Part model, mm, in its own coordinate system. Face numbers are marked on the shaded views. A direction names the side the tool comes from. Coordinates: 2 decimals unless noted, no trailing zeros. Write each loop counter-clockwise with the first axis right and the second up, starting at its lowest first coordinate (ties: lowest second). Pieces come first, ordered by that corner, then holes. Notation, with made-up numbers: M -6.5,33.25 L 6.5,33.25 A7 cw 6.5,45.25 Z; hole C 49,78.25 d3. An arc over 180 degrees is marked long. Use a Markdown table: item, result. Add a question column.
Q1. Slice it at B-B on y = 5. Write the cut outline in (x, z).
Q2. Slice it at D-D on x = 1.5. Write the cut outline in (y, z), then the cut area to 3 significant figures.
Q3. Tool access for the marked faces 1, 2 and 3: list every direction of +Z, -Z, +X, -X, +Y, -Y with a clear straight run to the whole face (end or side of a thin tool).
Q4. Pin check, flat tips, straight feed: pin 1 Ø2 at (x, y) = (16, 5) entering from +Z; pin 2 Ø11 at (x, y) = (14.5, 6) entering from -Z; pin 3 Ø2 at (x, z) = (8.5, 9.5) entering from +Y; pin 4 Ø5 at (y, z) = (6, 14) entering from +X. Stop position of each tip, or through.
Q5. Slice it at C-C on z = 7.25. Write the cut outline in (x, y).
Q6. Wall check: L1, parallel to Y at x = 24.5, z = 23.45; L2, parallel to Y at x = 21, z = 19.75; L3, parallel to X at y = 9, z = 18.5. Give the ranges that are in metal, low to high. Write a range as from..to.
Q7. Slice it at A-A on x = 16. Write the cut outline in (y, z).
from build123d import *

# Parameters (mm, degrees)
SKETCH1_W           = 12.5
SKETCH1_H           = 10
BOSS_EXTRUDE1_DEPTH = 10
SKETCH2_W           = 10
SKETCH2_H           = 10
BOSS_EXTRUDE2_DEPTH = 5
SKETCH3_R           = 3.75
BOSS_EXTRUDE3_DEPTH = 17
SKETCH4_W           = 4
SKETCH4_H           = 10
CUT_EXTRUDE1_DEPTH  = 11
SKETCH5_W           = 9.5
SKETCH5_H           = 10
BOSS_EXTRUDE4_DEPTH = 12.5
SKETCH6_W           = 5
SKETCH6_H           = 10
BOSS_EXTRUDE5_DEPTH = 30
SKETCH7_R           = 1.75
CUT_EXTRUDE2_DEPTH  = 23.5
SKETCH8_W           = 30
SKETCH8_H           = 5
CUT_EXTRUDE4_DEPTH  = 10
SKETCH10_W          = 9.5
SKETCH10_H          = 10
CUT_EXTRUDE6_DEPTH  = 3.49
SKETCH11_W          = 9.5
SKETCH11_H          = 10
BOSS_EXTRUDE6_DEPTH = 3.9
SKETCH12_W          = 4
SKETCH12_H          = 10
BOSS_EXTRUDE7_DEPTH = 20
SKETCH13_W          = 20
SKETCH13_H          = 0.09
CUT_EXTRUDE7_DEPTH  = 28
SKETCH14_R          = 1.75
CUT_EXTRUDE8_DEPTH  = 23.91
SKETCH15_W          = 29.5
SKETCH15_H          = 10
SKETCH15_R          = 1.75
BOSS_EXTRUDE8_DEPTH = 1
FILLET1_R           = 2


with BuildPart() as part:
    # Sketch1 → Boss-Extrude1 (new body)
    with BuildSketch(Plane.XY):
        with Locations((6.25, 5)):
            Rectangle(SKETCH1_W, SKETCH1_H)
    extrude(amount=BOSS_EXTRUDE1_DEPTH)

    # Sketch2 → Boss-Extrude2 (add)
    with BuildSketch(Plane.ZY):
        with Locations((5, 5)):
            Rectangle(SKETCH2_W, SKETCH2_H)
    extrude(amount=BOSS_EXTRUDE2_DEPTH)

    # Sketch3 → Boss-Extrude3 (add)
    with BuildSketch(Plane(origin=(0, 10, 0), x_dir=(1, 0, 0), z_dir=(0, 1, 0))):
        with Locations((3.75, -5)):
            Circle(SKETCH3_R)
    extrude(amount=BOSS_EXTRUDE3_DEPTH)

    # Sketch4 → Cut-Extrude1 (cut, through all)
    with BuildSketch(Plane(origin=(0, 10, 0), x_dir=(1, 0, 0), z_dir=(0, 1, 0))):
        with Locations((10.5, -5)):
            Rectangle(SKETCH4_W, SKETCH4_H)
        with Locations((-3, -5)):
            Rectangle(SKETCH4_W, SKETCH4_H)
    extrude(amount=-CUT_EXTRUDE1_DEPTH, mode=Mode.SUBTRACT)

    # Sketch5 → Boss-Extrude4 (add)
    with BuildSketch(Plane.XY.offset(10)):
        with Locations((3.75, 5)):
            Rectangle(SKETCH5_W, SKETCH5_H)
    extrude(amount=BOSS_EXTRUDE4_DEPTH)

    # Sketch6 → Boss-Extrude5 (add)
    with BuildSketch(Plane(origin=(8.5, 0, 0), x_dir=(0, 0, -1), z_dir=(1, 0, 0))):
        with Locations((-20, 5)):
            Rectangle(SKETCH6_W, SKETCH6_H)
    extrude(amount=BOSS_EXTRUDE5_DEPTH)

    # Sketch7 → Cut-Extrude2 (cut, through all)
    with BuildSketch(Plane.XY.offset(22.5)):
        with Locations((22.5, 5)):
            Circle(SKETCH7_R)
        with Locations((33.5, 5)):
            Circle(SKETCH7_R)
    extrude(amount=-CUT_EXTRUDE2_DEPTH, mode=Mode.SUBTRACT)

    # Sketch8 → Cut-Extrude4 (cut)
    with BuildSketch(Plane(origin=(0, 10, 0), x_dir=(1, 0, 0), z_dir=(0, 1, 0))):
        with Locations((23.5, -20)):
            Rectangle(SKETCH8_W, SKETCH8_H)
    extrude(amount=-CUT_EXTRUDE4_DEPTH, mode=Mode.SUBTRACT)

    # Sketch10 → Cut-Extrude6 (cut)
    with BuildSketch(Plane.XY.offset(22.5)):
        with Locations((3.75, 5)):
            Rectangle(SKETCH10_W, SKETCH10_H)
    extrude(amount=-CUT_EXTRUDE6_DEPTH, mode=Mode.SUBTRACT)

    # Sketch11 → Boss-Extrude6 (add)
    with BuildSketch(Plane.XY.offset(19.01)):
        with Locations((3.75, 5)):
            Rectangle(SKETCH11_W, SKETCH11_H)
    extrude(amount=BOSS_EXTRUDE6_DEPTH)

    # Sketch12 → Boss-Extrude7 (add)
    with BuildSketch(Plane(origin=(8.5, 0, 0), x_dir=(0, 0, -1), z_dir=(1, 0, 0))):
        with Locations((-20.91, 5)):
            Rectangle(SKETCH12_W, SKETCH12_H)
    extrude(amount=BOSS_EXTRUDE7_DEPTH)

    # Sketch13 → Cut-Extrude7 (cut, through all)
    with BuildSketch(Plane(origin=(0, 0, 0), x_dir=(-1, 0, 0), z_dir=(0, -1, 0))):
        with Locations((-18.5, -18.955)):
            Rectangle(SKETCH13_W, SKETCH13_H)
    extrude(amount=-CUT_EXTRUDE7_DEPTH, mode=Mode.SUBTRACT)

    # Sketch14 → Cut-Extrude8 (cut, through all)
    with BuildSketch(Plane.XY.offset(22.91)):
        with Locations((16, 5)):
            Circle(SKETCH14_R)
        with Locations((24.5, 5)):
            Circle(SKETCH14_R)
    extrude(amount=-CUT_EXTRUDE8_DEPTH, mode=Mode.SUBTRACT)

    # Sketch15 → Boss-Extrude8 (add)
    with BuildSketch(Plane.XY.offset(22.91)):
        with Locations((13.75, 5)):
            Rectangle(SKETCH15_W, SKETCH15_H)
        with Locations((24.5, 5)):
            Circle(SKETCH15_R, mode=Mode.SUBTRACT)
        with Locations((16, 5)):
            Circle(SKETCH15_R, mode=Mode.SUBTRACT)
    extrude(amount=BOSS_EXTRUDE8_DEPTH)

    # Fillet1
    fillet1_edges = [part.edges().sort_by_distance(p)[0] for p in [
        (-1, 5, 23.91),
    ]]
    fillet(fillet1_edges, radius=FILLET1_R)


solid = part.part
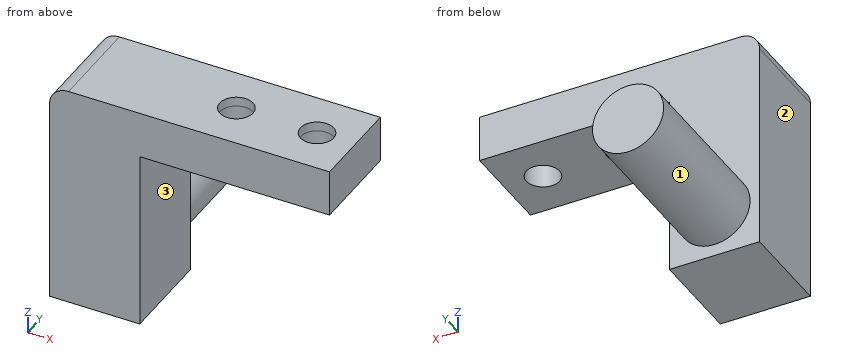
Recorded:
| question | item | result |
|---|---|---|
| 1 | outline | M -1,0 L 8.5,0 L 8.5,19 L 14.25,19 L 14.25,23.91 L 1,23.91 A2 ccw -1,21.91 Z; M 17.75,19 L 22.75,19 L 22.75,23.91 L 17.75,23.91 Z; M 26.25,19 L 28.5,19 L 28.5,23.91 L 26.25,23.91 Z |
| 2 | outline | M 0,0 L 10,0 L 10,2 L 27,2 L 27,8 L 10,8 L 10,23.91 L 0,23.91 Z |
| 2 | area | 341 mm² |
| 3 | face 1 | +Y |
| 3 | face 2 | +Z, -Z, -X, +Y, -Y |
| 3 | face 3 | -Z, +X, +Y, -Y |
| 4 | pin 1 | through |
| 4 | pin 2 | z = 19 |
| 4 | pin 3 | y = 10 |
| 4 | pin 4 | x = 8.5 |
| 5 | outline | M -1,0 L 8.5,0 L 8.5,10 L 6.75,10 L 6.75,27 L 0.75,27 L 0.75,10 L -1,10 Z |
| 6 | L1 | 0..3.25, 6.75..10 |
| 6 | L2 | 0..10 |
| 6 | L3 | -1..8.5 |
| 7 | outline | M 0,19 L 3.25,19 L 3.25,23.91 L 0,23.91 Z; M 6.75,19 L 10,19 L 10,23.91 L 6.75,23.91 Z |
